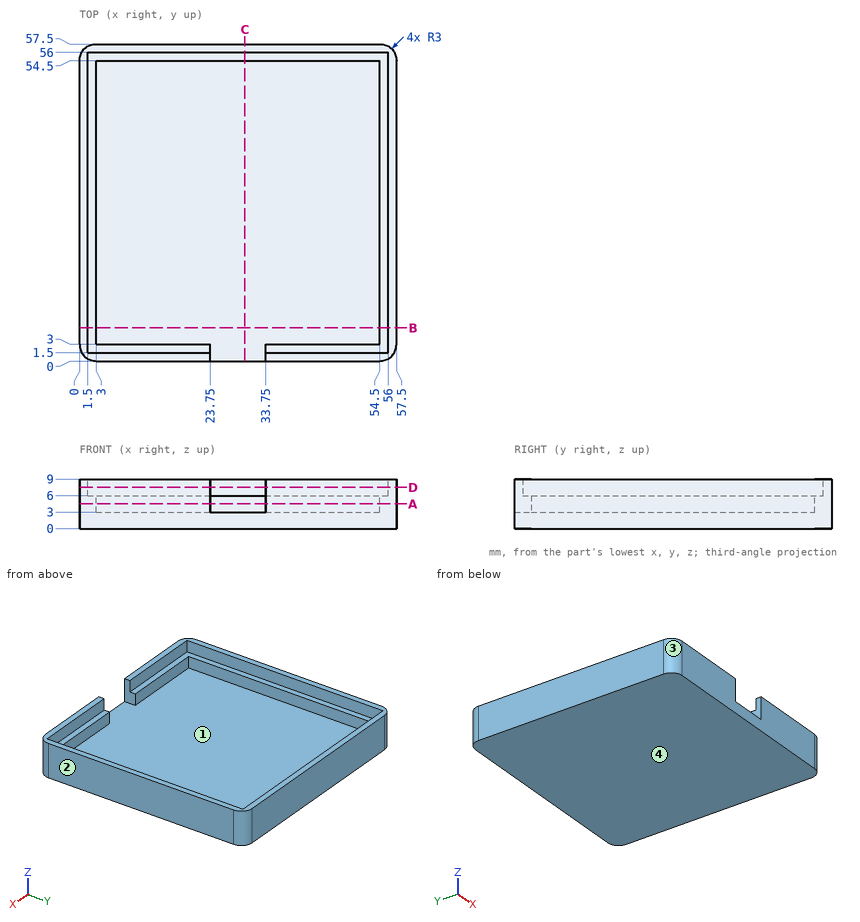
Design review of the part shown in the three views and the two pictorial views. Dimensions are in mm from the part's minimum x, y and z. Round coordinates to 2 decimals unless told otherwise and drop trailing zeros. Loops run counter-clockwise (first coordinate to the right, second up) from the corner with the lowest first, then second, coordinate; pieces in that order, holes last. Notation, with made-up numbers: (1.25, 73) -> (33.25, 73) arc R15 cw to (33.25, 85) -> close; hole circle Ø3 at (28.25, -18). An arc over 180 degrees is marked (long way). Use one line per item in the form item = value. Start each with the question number.
Q1. Wall thickness on line 1 along X through (y, z) = (53, 4.25); line 2 along X through (y, z) = (46, 6.5): over which ranges is each line inside the solid? List them lowest first. Write a range as [from, to].
Q2. For pin 1 Ø1.5 at (y, z) = (1.5, 6.5) entering from -X; pin 2 Ø3.5 at (x, z) = (26, 8) entering from -Y; pin 3 Ø3.5 at (x, z) = (31, 4.5) entering from -Y; pin 4 Ø16.5 at (x, y) = (20.5, 39.5) entering from +Z, all flat-tipped, find the tip position at first contact; note any pin that passes through.
Q3. We need section D-D on z = 7.5. Give the boundary of the cut face in (x, y), then the cut area to 3 significant figures.
Q4. We need section B-B on y = 6. Give the boundary of the cut face in (x, z), then the cut area to 4 significant figures.
Q5. Draft analysis for pull direction X (two halves, no side actions). For the marked faces 1, 2, 3 and 4, state which applies: +X half, -X half, draft (parallel to the pull), parting line (faces both ways), or undercut.
Q6. We need section C-C on x = 30. Give the boundary of the cut face in (y, z).
Q7. We need section A-A on z = 4.5. Give the boundary of the cut face in (x, y), then the cut area to 3 significant figures.
Calculated:
q1.line_1 = [0, 3], [54.5, 57.5]
q1.line_2 = [0, 1.5], [56, 57.5]
q2.pin_1 = 0.1
q2.pin_2 = 56
q2.pin_3 = 0
q2.pin_4 = 3
q3.outline = (0, 3) arc R3 ccw to (3, 0) -> (23.75, 0) -> (23.75, 1.5) -> (1.5, 1.5) -> (1.5, 56) -> (56, 56) -> (56, 1.5) -> (33.75, 1.5) -> (33.75, 0) -> (54.5, 0) arc R3 ccw to (57.5, 3) -> (57.5, 54.5) arc R3 ccw to (54.5, 57.5) -> (3, 57.5) arc R3 ccw to (0, 54.5) -> close
q3.area = 313 mm²
q4.outline = (0, 0) -> (57.5, 0) -> (57.5, 9) -> (56, 9) -> (56, 6) -> (54.5, 6) -> (54.5, 3) -> (3, 3) -> (3, 6) -> (1.5, 6) -> (1.5, 9) -> (0, 9) -> close
q4.area = 199.5 mm²
q5.face_1 = undercut
q5.face_2 = +X half
q5.face_3 = -X half
q5.face_4 = draft
q6.outline = (0, 0) -> (57.5, 0) -> (57.5, 9) -> (56, 9) -> (56, 6) -> (54.5, 6) -> (54.5, 3) -> (0, 3) -> close
q7.outline = (0, 3) arc R3 ccw to (3, 0) -> (23.75, 0) -> (23.75, 3) -> (3, 3) -> (3, 54.5) -> (54.5, 54.5) -> (54.5, 3) -> (33.75, 3) -> (33.75, 0) -> (54.5, 0) arc R3 ccw to (57.5, 3) -> (57.5, 54.5) arc R3 ccw to (54.5, 57.5) -> (3, 57.5) arc R3 ccw to (0, 54.5) -> close
q7.area = 616 mm²
